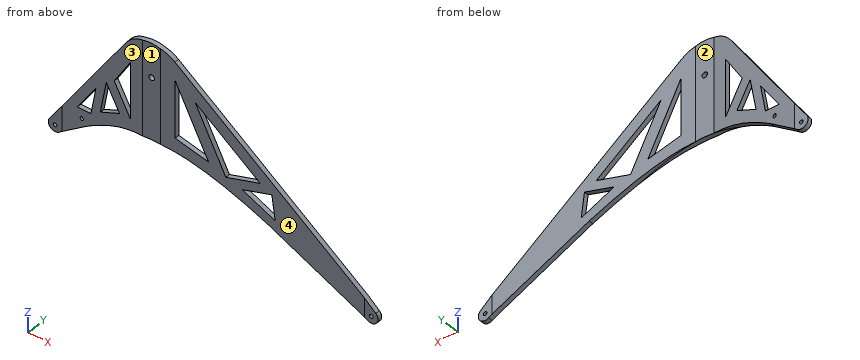
```python
from build123d import *

# Parameters (mm, degrees)
F1_W     = 30
F1_H     = 10
F2_DEPTH = 340
F3_DEPTH = 100
F5_DEPTH = 76
F6_R     = 4
F6_R_2   = 6
F7_DEPTH = 66


with BuildPart() as f2:
    # F1 (on Top) → F2 (new body)
    with BuildSketch(Plane.XY):
        Polygon((0, 0), (-20, 0), (-20, -10), (20, -10), (20, 0), align=None)
        Polygon((-20, -10), (-20, 0), (-223.64854, 33), (-223.64854, 23), align=None)
        with Locations((-238.64854, 28)):
            Rectangle(F1_W, F1_H)
        Polygon((442.00493, 33), (20, 0), (20, -10), (442.00493, 23), align=None)
        with Locations((457.00493, 28)):
            Rectangle(F1_W, F1_H)
    extrude(amount=-F2_DEPTH)

    # F1 (on Top) → F3 (join)
    with BuildSketch(Plane.XY):
        Polygon((0, 0), (-20, 0), (-20, -10), (20, -10), (20, 0), align=None)
        Polygon((-20, -10), (-20, 0), (-223.64854, 33), (-223.64854, 23), align=None)
        with Locations((-238.64854, 28)):
            Rectangle(F1_W, F1_H)
        Polygon((442.00493, 33), (20, 0), (20, -10), (442.00493, 23), align=None)
        with Locations((457.00493, 28)):
            Rectangle(F1_W, F1_H)
    extrude(amount=F3_DEPTH)

    # F4 (on Front) → F5 (intersect, symmetric)
    with BuildSketch(Plane.XZ):
        with BuildLine():
            ThreePointArc((-250.9718022583, -230.0965111685), (-249.006915225, -249.4976876834), (-229.5356153331, -250.563010045))
            ThreePointArc((-229.5356153331, -250.563010045), (-225.2006047987, -245.2933166844), (-223.6485386505, -238.6485386505))
            ThreePointArc((-223.6485386505, -238.6485386505), (-234.1679669301, -224.3333552056), (-250.9718022583, -230.0965111685))
        make_face()
        with BuildLine():
            add(Edge.make_bspline(
                [(-229.5356153331, -250.563010045), (-208.7207010553, -234.6424785008), (-187.0701685552, -217.0301430269), (-164.0481391717, -200.4741451059)],
                knots=[0, 0, 0, 0, 0.1373195068, 0.1373195068, 0.1373195068, 0.1373195068], degree=3))
            Line((-229.5356153331, -250.563010045), (-164.0481391717, -200.4741451059))
        make_face()
        with BuildLine():
            ThreePointArc((-223.6485386505, -238.6485386505), (-225.2006047987, -245.2933166844), (-229.5356153331, -250.563010045))
            add(Edge.make_bspline(
                [(-229.5356153331, -250.563010045), (-208.7207010553, -234.6424785008), (-187.0701685552, -217.0301430269), (-164.0481391717, -200.4741451059)],
                knots=[0, 0, 0, 0, 0.1373195068, 0.1373195068, 0.1373195068, 0.1373195068], degree=3))
            Line((-164.0481391717, -200.4741451059), (0, -75))
            ThreePointArc((0, -75), (-66.4530293795, -34.7706037666), (-61.6163187638, 42.7601363655))
            Line((-61.6163187638, 42.7601363655), (-250.9718022583, -230.0965111685))
            ThreePointArc((-250.9718022583, -230.0965111685), (-234.1679669301, -224.3333552056), (-223.6485386505, -238.6485386505))
        make_face()
        with BuildLine():
            Line((0, -75), (-164.0481391717, -200.4741451059))
            add(Edge.make_bspline(
                [(-164.0481391717, -200.4741451059), (-116.7152354778, -166.4352929221), (-4.1014041633, -103.751655246), (155.4809175381, -168.4276528716), (240.7432263876, -213.1721002441)],
                knots=[0.1373195068, 0.1373195068, 0.1373195068, 0.1373195068, 0.4196460942, 0.7357326781, 0.7357326781, 0.7357326781, 0.7357326781], degree=3))
            Line((240.7432263876, -213.1721002441), (0, -75))
        make_face()
        with BuildLine():
            ThreePointArc((49.3759786376, 56.4536334843), (-9.1833788682, 74.4356470555), (-61.6163187638, 42.7601363655))
            ThreePointArc((-61.6163187638, 42.7601363655), (-66.4530293795, -34.7706037666), (0, -75))
            ThreePointArc((0, -75), (53.033008589, -53.033008589), (75, 0))
            ThreePointArc((75, 0), (68.2942105812, 30.9983999763), (49.3759786376, 56.4536334843))
        make_face()
        with BuildLine():
            ThreePointArc((75, 0), (53.033008589, -53.033008589), (0, -75))
            Line((0, -75), (240.7432263876, -213.1721002441))
            add(Edge.make_bspline(
                [(240.7432263876, -213.1721002441), (312.0276249141, -250.5811390256), (383.9898125383, -295.3870059685), (449.5382273905, -333.0078449167)],
                knots=[0.7357326781, 0.7357326781, 0.7357326781, 0.7357326781, 1, 1, 1, 1], degree=3))
            ThreePointArc((449.5382273905, -333.0078449167), (444.7952538382, -311.2848606652), (466.8801220688, -308.7075678715))
            Line((466.8801220688, -308.7075678715), (49.3759786376, 56.4536334843))
            ThreePointArc((49.3759786376, 56.4536334843), (68.2942105812, 30.9983999763), (75, 0))
        make_face()
        with BuildLine():
            add(Edge.make_bspline(
                [(240.7432263876, -213.1721002441), (312.0276249141, -250.5811390256), (383.9898125383, -295.3870059685), (449.5382273905, -333.0078449167)],
                knots=[0.7357326781, 0.7357326781, 0.7357326781, 0.7357326781, 1, 1, 1, 1], degree=3))
            Line((240.7432263876, -213.1721002441), (449.5382273905, -333.0078449167))
        make_face()
        with BuildLine():
            ThreePointArc((466.8801220688, -308.7075678715), (444.7952538382, -311.2848606652), (449.5382273905, -333.0078449167))
            ThreePointArc((449.5382273905, -333.0078449167), (464.521558007, -332.979057912), (472.0049255088, -319.9982938402))
            ThreePointArc((472.0049255088, -319.9982938402), (470.6637678536, -313.7986143485), (466.8801220688, -308.7075678715))
        make_face()
    extrude(amount=F5_DEPTH, both=True, mode=Mode.INTERSECT)

    # F6 (on face) → F7 (cut, symmetric)
    with BuildSketch(Plane.XZ.offset(10)):
        Polygon((-50, -118.8666767037), (-50, 6.8798678522), (-91.5673471808, -58.5868135927), align=None)
        Polygon((-126.4676634488, -146.9804479722), (-78.2616292159, -121.9207695), (-111.7079214913, -73.417844568), align=None)
        Polygon((-150.4108945671, -164.6469025725), (-137.8857839916, -102.2217094685), (-184.8640607304, -169.9162639715), align=None)
        Polygon((50, 16.0521292518), (50, -109.3419641256), (118.974648416, -131.2328726053), align=None)
        Polygon((225.9725652657, -131.215947327), (91.4881845235, -13.5920175816), (154.9125586599, -149.0252423531), align=None)
        Polygon((250.1992884028, -145.7627206944), (188.8613105429, -161.1354485647), (256.9922346805, -199.3553946004), align=None)
        with Locations((-238.6485386505, -238.6485386505)):
            Circle(F6_R)
        with Locations((457.0049255088, -319.9982938402)):
            Circle(F6_R)
        Circle(F6_R_2)
        with Locations((-173.5450253277, -188.5422087565)):
            Circle(F6_R)
    extrude(amount=F7_DEPTH, both=True, mode=Mode.SUBTRACT)


solid = f2.part
```
Verification items for the finished model (mm, model axes). Face numbers are marked on the shaded views. Round coordinates to 2 decimals unless told otherwise and drop trailing zeros. Write each loop counter-clockwise with the first axis right and the second up, starting at its lowest first coordinate (ties: lowest second). Pieces come first, ordered by that corner, then holes. Notation, with made-up numbers: (-40, 27.25) -> (-28, 27.25) arc R21 ccw to (-28, 44.25) -> close; hole circle Ø6 at (81, 75.5). An arc over 180 degrees is marked (long way). Write each question's results on one line, items separated by ' | '.
Q1. Draft check along X on the marked faces 1, 2, 3 and 4. Enter one of: released by +X, released by -X, zero draft, split by the parting line, or undercut.
Derived:
face 1: zero draft | face 2: undercut | face 3: released by -X | face 4: released by +X
Q2. Thickness scan on probe 1 along Y at (x, z) = (12, -55.5); probe 2 along Y at (x, z) = (345.5, -229.5); probe 3 along Z at (x, y) = (-92.5, 8). Record the ranges inside material, lowest first.
Derived:
probe 1: y = -10 to 0 | probe 2: y = 15.45 to 25.45 | probe 3: z = -157.7 to -129.32, -101.27 to -1.74
Q3. Sectioned sample at A-A, the plane z = -48. Record the boundary of the cut face in (x, y), and give its area (3 significant figures).
Derived:
outline: (-124.6, 6.95) -> (-84.85, 0.51) -> (-84.85, 10.51) -> (-124.6, 16.95) -> close; (-50, -5.14) -> (-20, -10) -> (20, -10) -> (50, -7.65) -> (50, 2.35) -> (20, 0) -> (-20, 0) -> (-50, 4.86) -> close; (80, -5.31) -> (107.6, -3.15) -> (107.6, 6.85) -> (80, 4.69) -> close; (130.83, -1.33) -> (168.8, 1.64) -> (168.8, 11.64) -> (130.83, 8.67) -> close | area: 2,050 mm²
Q4. Sectioned sample at C-C, the plane x = -209. Record the boundary of the cut face in (y, z).
Derived:
outline: (20.63, -234.86) -> (30.63, -234.86) -> (30.63, -169.62) -> (20.63, -169.62) -> close
Q5. Go/stop test with flat-tipped pins: pin 1 Ø20 at (x, z) = (-6, -29.5) entering from +Y; pin 2 Ø9 at (x, z) = (-238.65, -238.65) entering from -Y; pin 3 Ø13 at (x, z) = (-173.55, -188.54) entering from -Y. Record where each tip stops, or that it passes through.
Derived:
pin 1: stops at y = 0 | pin 2: stops at y = 23 | pin 3: stops at y = 13.83
Q6. Sectioned sample at D-D, the plane x = 378. Record the boundary of the cut face in (y, z), and give its area (3 significant figures).
Derived:
outline: (17.99, -291.95) -> (27.99, -291.95) -> (27.99, -230.97) -> (17.99, -230.97) -> close | area: 610 mm²
Q7. Sectioned sample at B-B, the plane x = 109.5. Give the number of separate pieces and of enclosed holes in the cut face, and give its area (3 significant figures).
Derived:
separate pieces: 3 | enclosed holes: 0 | area: 1,190 mm²
